Source: three-view drawing plus pictorial views. Frame: mm from the lowest corner of the part. Round coordinates to 2 decimals unless told otherwise and drop trailing zeros. Loops run counter-clockwise (first coordinate to the right, second up) from the corner with the lowest first, then second, coordinate; pieces in that order, holes last. Notation, with made-up numbers: (-26.75, 0.25) -> (-16.75, 0.25) arc R8 cw to (-16.75, 11.25) -> close; hole circle Ø8 at (-23, 82.5). An arc over 180 degrees is marked (long way). Put each result on its own line as item: value. Start each with the question number.
1. Draft query along X for the marked faces 1, 2, 3 and 4. Return one class per face: pulls with the +X half, pulls with the -X half, needs draft (parallel to the pull), parting line crosses it, or undercut.
2. Material intervals for L1, parallel to Y at x = 19.05, z = 18.5; L2, parallel to Z at x = 16.5, y = 7, sorted ascending.
3. Contact query for a flat-ended pin moving along its axis: pin 1 (8 mm diameter, centred on x = 17, y = 13, fed in from +Z). Output: stop coordinate, or through.
4. Cut plane A-A (y = 19.05). Return the cut outline in (x, z), then the cut area to 3 significant figures.
5. Cut plane C-C (z = 19.5). Return the cut outline in (x, y), then the cut area to 3 significant figures.
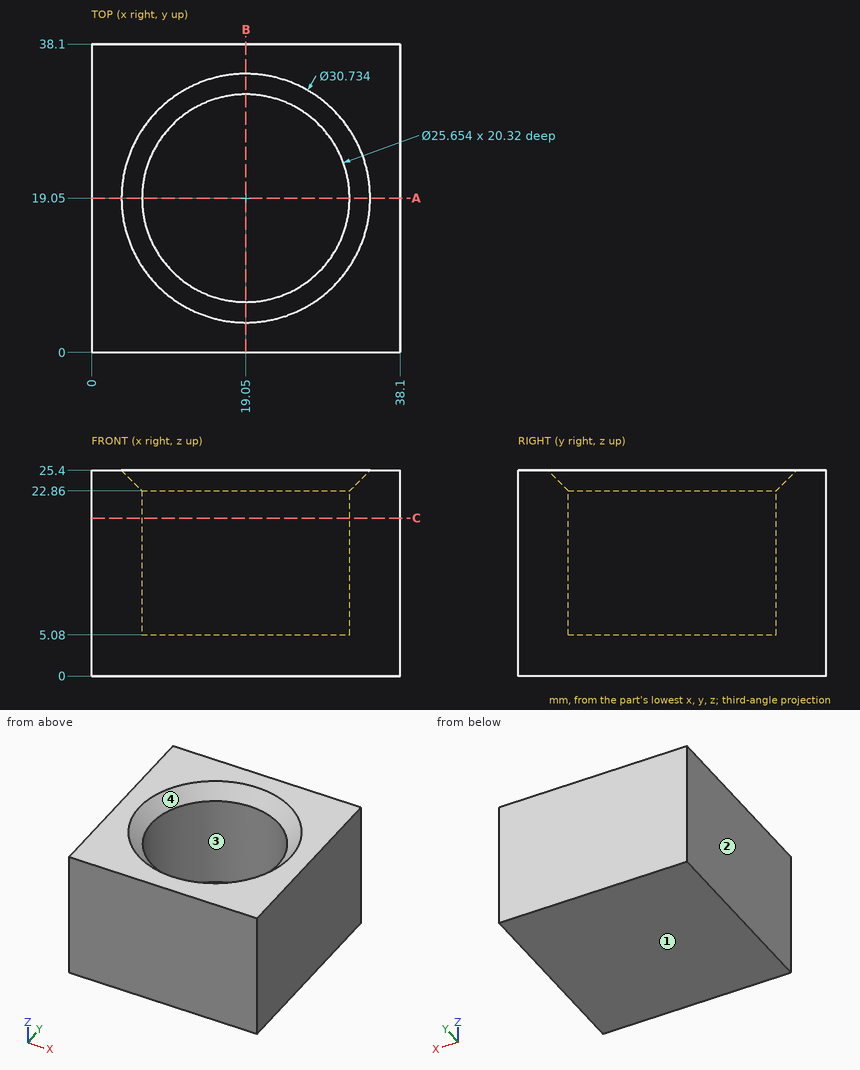
Solution:
1. face 1: needs draft
1. face 2: pulls with the -X half
1. face 3: undercut
1. face 4: undercut
2. L1: y = 0 to 6.22, 31.88 to 38.1
2. L2: z = 0 to 5.08
3. pin 1: stops at z = 5.08
4. outline: (0, 0) -> (38.1, 0) -> (38.1, 25.4) -> (34.42, 25.4) -> (31.88, 22.86) -> (31.88, 5.08) -> (6.22, 5.08) -> (6.22, 22.86) -> (3.68, 25.4) -> (0, 25.4) -> close
4. area: 440 mm^2
5. outline: (0, 0) -> (38.1, 0) -> (38.1, 38.1) -> (0, 38.1) -> close; hole circle Ø25.65 at (19.05, 19.05)
5. area: 935 mm^2
